Verification items for the finished model (mm, model axes). Face numbers are marked on the shaded views. A direction names the side the tool comes from. Coordinates: 2 decimals unless noted, no trailing zeros. Loops run counter-clockwise (first coordinate to the right, second up) from the corner with the lowest first, then second, coordinate; pieces in that order, holes last. Notation, with made-up numbers: (70, 76) -> (122, 76) arc R36 ccw to (122, 114) -> close; hole circle Ø6 at (86.5, 33.25). An arc over 180 degrees is marked (long way). Use CSV: the item, a comma, the result in double quotes. Start each with the question number.
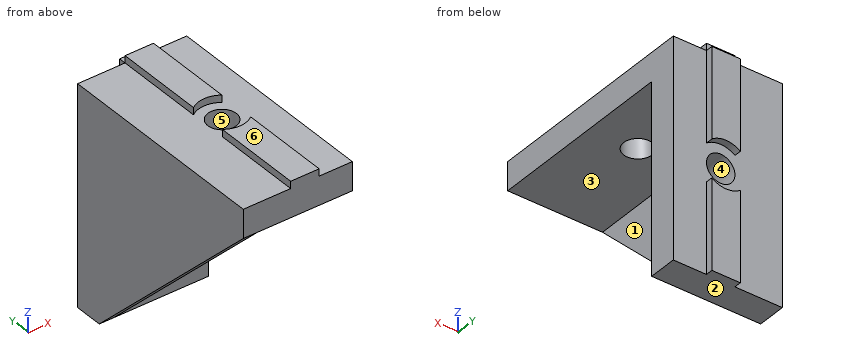
Autodesk Inventor part; units mm, degrees
ref_plane "YZ Plane" through (0, 0, 0) normal (1, 0, 0) x (0, 1, 0)
ref_plane "XZ Plane" through (0, 0, 0) normal (0, 1, 0) x (-1, 0, 0)
ref_plane "XY Plane" through (0, 0, 0) normal (0, 0, 1) x (1, 0, 0)
sketch "Sketch1" plane through (0, 0, 0) normal (0, 0, 1) x (1, 0, 0)
  line L0 (0, 6) -> (0, -40)
  line L1 (-20, 6) -> (-20, -40)
  line L2 (-20, 6) -> (0, 6)
  line L3 (-20, -40) -> (0, -40)
  point P0 (0, 0)
  dimension "d6" = 20
  dimension "d10" = 6
extrude "Extrusion1" add sketch "Sketch1" against normal blind 6
sketch "Sketch2" plane through (0, 0, -6) normal (0, 0, -1) x (-1, 0, 0)
  line L0 (20, -40) -> (20, 6)
  line L1 (0, 6) -> (0, -40)
  line L2 (20, 6) -> (0, 6)
  line L3 (0, 6) -> (0, 0)
  line L4 (0, 0) -> (20, 0)
  line L5 (20, 0) -> (20, 6)
  point P0 (0, 0)
  dimension "d13" = 6
extrude "Extrusion2" add sketch "Sketch2" along normal blind 40
sketch "Sketch3" plane through (0, 0, 0) normal (0, 0, 1) x (1, 0, 0)
  line L0 (0, 6) -> (-20, 6)
  line L1 (-13, 6) -> (-13, -40)
  line L2 (-20, 6) -> (-20, -40)
  line L3 (-7, 6) -> (-7, -40)
  line L4 (0, -40) -> (-20, -40)
  line L5 (-13, 6) -> (-7, 6)
  line L6 (-13, -40) -> (-7, -40)
  point P0 (0, 0)
  dimension "d16" = 7
  dimension "d17" = 6
extrude "Extrusion3" add sketch "Sketch3" along normal blind 1.5 contours L3 L4 L1 L0
sketch "Sketch4" plane through (-20, 6, -46) normal (0, 1, 0) x (1, 0, 0)
  line L0 (20, -46) -> (13, -46)
  line L1 (13, -46) -> (13, 0)
  line L2 (20, 0) -> (0, 0)
  line L3 (7, -46) -> (7, -47.5)
  line L4 (7, -46) -> (7, 0)
  line L5 (7, 0) -> (13, 0)
  line L6 (7, -46) -> (13, -46)
extrude "Extrusion4" add sketch "Sketch4" along normal blind 1.5
sketch "Sketch5" plane through (-20, 7.5, -46) normal (0, 1, 0) x (1, 0, 0)
  line L0 (20, -46) -> (20, 0)
  line L1 (0, 0) -> (7, 0)
  point P0 (10, -23)
  dimension "d22" = 10
  dimension "d23" = 23
hole "Hole1" at (-10, 7.5, -23) direction (0, -1, 0) diameter 6 end through all counterbore diameter 10 counterbore depth 1.5
sketch "Sketch6" plane through (0, 0, 1.5) normal (0, 0, 1) x (1, 0, 0)
  line L0 (-7, -40) -> (0, -40)
  line L1 (0, -40) -> (0, 6)
  point P0 (0, 0)
  point P1 (-10, -17)
  dimension "d31" = 23
  dimension "d32" = 10
hole "Hole2" at (-10, -17, 1.5) direction (0, 0, -1) diameter 6 end through all counterbore diameter 10 counterbore depth 1.5
sketch "Sketch7" plane through (-20, -40, 0) normal (-1, 0, 0) x (0, 0, 1)
  line L0 (0, 0) -> (0, 46)
  line L1 (0, 46) -> (-46, 46)
  line L2 (0, 0) -> (0, 46)
  line L3 (-46, 46) -> (-46, 40)
  line L4 (0, 46) -> (-46, 46)
  line L5 (-46, 46) -> (-46, 40)
  line L6 (0, 0) -> (-6, 0)
  line L7 (-46, 40) -> (-6, 0)
  line L8 (-6, 0) -> (0, 0)
  point P0 (0, 40)
extrude "Extrusion5" add sketch "Sketch7" along normal blind 3
properties part number "Estrutura - SuporteCanto"
1. Release check for a two-part mould opening along Z. For the marked faces 3, 4, 5 and 6 record: released by +Z, released by -Z, zero draft, split by the parting line, or undercut.
2. Set-up check for the marked faces 1 and 2: record each of +Z, -Z, +X, -X, +Y, -Y from which the full face is reachable in a straight line by a thin tool's end or side.
3. Cross-section at B-B, the plane x = -10. Record the boundary of the cut face in (y, z), plus the area to 3 significant figures.
4. Scan lines: line 1 (X direction, y = -17, z = -3); line 2 (Y direction, x = -10, z = -2.25); line 3 (Y direction, x = -2, z = -26). Record each from-to range of solid material in increasing order.
5. Cross-section at C-C, the plane y = 2. Record the boundary of the cut face in (x, z).
6. Depth check by flat-ended pin: pin 1 (9.5 mm diameter, centred on x = -10, z = -23, fed in from +Y); pin 2 (0.8 mm diameter, centred on y = 6.5, z = -9.5, fed in from +X); pin 3 (10 mm diameter, centred on x = -14, y = -10.5, fed in from -Z); pin 4 (7 mm diameter, centred on x = -10.5, z = -24.5, fed in from +Y). Enter the tip coordinate at first touch or a pass-through.
7. Cross-section at A-A, the plane z = -23. Record the boundary of the cut face in (x, y), plus the area to 3 significant figures.
8. Cross-section at D-D, the plane y = -18.5. Record the boundary of the cut face in (x, z), plus the area to 3 significant figures.
Solution:
1,face 3,"released by -Z"
1,face 4,"undercut"
1,face 5,"zero draft"
1,face 6,"released by +Z"
2,face 1,"-Z, +X, -Y"
2,face 2,"-Z, +X, -X, +Y, -Y"
3,outline,"(-40, -6) -> (-20, -6) -> (-20, 0) -> (-22, 0) -> (-22, 1.5) -> (-40, 1.5) -> close; (-14, -6) -> (0, -6) -> (0, -20) -> (6, -20) -> (6, -18) -> (7.5, -18) -> (7.5, 0) -> (6, 0) -> (6, 1.5) -> (-12, 1.5) -> (-12, 0) -> (-14, 0) -> close; (0, -46) -> (7.5, -46) -> (7.5, -28) -> (6, -28) -> (6, -26) -> (0, -26) -> close"
3,area,"552 mm2"
4,line 1,"x = -23 to -13, -7 to 0"
4,line 2,"y = -40 to -20, -14 to 7.5"
4,line 3,"y = 0 to 6"
5,outline,"(-23, -46) -> (0, -46) -> (0, 0) -> (-7, 0) -> (-7, 1.5) -> (-13, 1.5) -> (-13, 0) -> (-23, 0) -> close; hole circle Ø6 at (-10, -23)"
6,pin 1,"stops at y = 6"
6,pin 2,"stops at x = -7"
6,pin 3,"stops at z = -6"
6,pin 4,"stops at y = 7.5"
7,outline,"(-23, -23) -> (-20, -23) -> (-20, 0) -> (-13, 0) -> (-13, 6) -> (-23, 6) -> close; (-7, 0) -> (0, 0) -> (0, 6) -> (-7, 6) -> close"
7,area,"171 mm2"
8,outline,"(-23, -27.5) -> (-20, -27.5) -> (-20, -6) -> (-12.6, -6) -> (-12.6, 0) -> (-23, 0) -> close; (-7.4, -6) -> (0, -6) -> (0, 0) -> (-7.4, 0) -> close"
8,area,"171 mm2"
